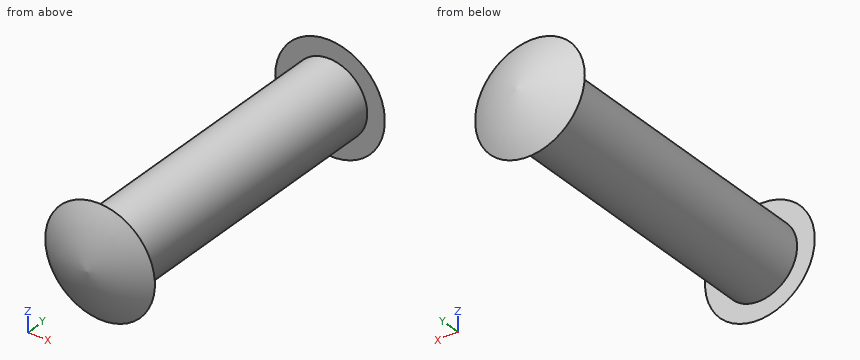
from build123d import *

# Parameters (mm, degrees)
SKETCH1_R           = 3.175
BOSS_EXTRUDE1_DEPTH = 12.7889


with BuildPart() as part:
    # Sketch1 → Boss-Extrude1 (new body, symmetric)
    with BuildSketch(Plane(origin=(0, 0, 0), x_dir=(1, 0, 0), z_dir=(0, 1, 0))):
        Circle(SKETCH1_R)
    extrude(amount=BOSS_EXTRUDE1_DEPTH, both=True)

    # Sketch3 → Revolve1 (revolve)
    with BuildSketch(Plane.XY):
        with BuildLine():
            Line((0, 12.7889), (-4.68122, 12.7889))
            add(Edge.make_bspline(
                [(-4.68122, 12.7889), (-2.485687352, 14.067463283), (0, 14.3129)],
                knots=[0, 0, 0, 1, 1, 1], degree=2))
            Line((0, 14.3129), (0, 12.7889))
        make_face()
    revolve1 = revolve(axis=Axis((0, 12.7889, 0), (0, 1, 0)))

    # Mirror1: Revolve1 across plane
    add(revolve1.mirror(Plane.ZX))


solid = part.part
Build history of the part. All positions in model axes, mm. Coordinates: 2 decimals unless noted, no trailing zeros. Order: outer loops, then holes, each group sorted by start corner. A loop starts at its lowest first (then second) coordinate and runs counter-clockwise, first axis right, second up. Notation, with made-up numbers: (44.5, -40) - (76.5, -40) arc R22 ccw to (76.5, -4) - close; hole circle Ø7 at (14.25, 45). An arc over 180 degrees is marked (long way). Put each result on its own line as item: value.
1. Drop flat-ended pins along their axis: P1, Ø2, axis at x = 3.5, z = -0.5, coming from the +Y side; P2, Ø3, axis at y = 3.5, z = 3, coming from the -X side; P3, Ø4, axis at x = 3, z = 0, coming from the +Y side. Give the stop position or say it passes through.
Answer sheet:
P1: stops at y = 13.77
P2: stops at x = -2.8
P3: stops at y = 14.17
2. Saw through at A-A (y = 12.25). Write the cut outline in (x, z) (3 decimals).
Answer sheet:
outline: circle Ø6.35 at (0, 0)
3. Probe line 1 along Y through (x, z) = (4, -0.5); line 2 along X through (y, z) = (3.25, 0) (3 decimals); line 3 along Y through (x, z) = (3.5, 2.5). List the from-to ranges inside material, lowest first. Write a range as [from, to].
Answer sheet:
line 1: y = [-13.14, -12.79], [12.79, 13.14]
line 2: x = [-3.175, 3.175]
line 3: y = [-13, -12.79], [12.79, 13]
